```python
from build123d import *

# Parameters (mm, degrees)
SKETCH1_W           = 16
SKETCH1_H           = 20
BOSS_EXTRUDE1_DEPTH = 1.8
SKETCH2_W           = 16
SKETCH2_H           = 18.2
BOSS_EXTRUDE2_DEPTH = 1.8
SKETCH3_R           = 2.6
CUT_EXTRUDE1_DEPTH  = 1.8
SKETCH4_R           = 2.6
CUT_EXTRUDE2_DEPTH  = 1.8
FILLET1_R           = 2


with BuildPart() as part:
    # Sketch1 → Boss-Extrude1 (new body)
    with BuildSketch(Plane.XY):
        with Locations((8, 10)):
            Rectangle(SKETCH1_W, SKETCH1_H)
    extrude(amount=BOSS_EXTRUDE1_DEPTH)

    # Sketch2 → Boss-Extrude2 (add)
    with BuildSketch(Plane.XZ):
        with Locations((8, 10.9)):
            Rectangle(SKETCH2_W, SKETCH2_H)
    extrude(amount=-BOSS_EXTRUDE2_DEPTH)

    # Sketch3 → Cut-Extrude1 (cut)
    with BuildSketch(Plane.XY.offset(1.8)):
        with Locations((8, 10.8)):
            Circle(SKETCH3_R)
    extrude(amount=-CUT_EXTRUDE1_DEPTH, mode=Mode.SUBTRACT)

    # Sketch4 → Cut-Extrude2 (cut)
    with BuildSketch(Plane(origin=(0, 1.8, 0), x_dir=(1, 0, 0), z_dir=(0, 1, 0))):
        with Locations(Location((8, -10.8, 0), (0, 0, 270))):
            Circle(SKETCH4_R)
    extrude(amount=-CUT_EXTRUDE2_DEPTH, mode=Mode.SUBTRACT)

    # Fillet1
    fillet1_edges = [part.edges().sort_by_distance(p)[0] for p in [
        (8, 1.8, 1.8),
    ]]
    fillet(fillet1_edges, radius=FILLET1_R)


solid = part.part
```
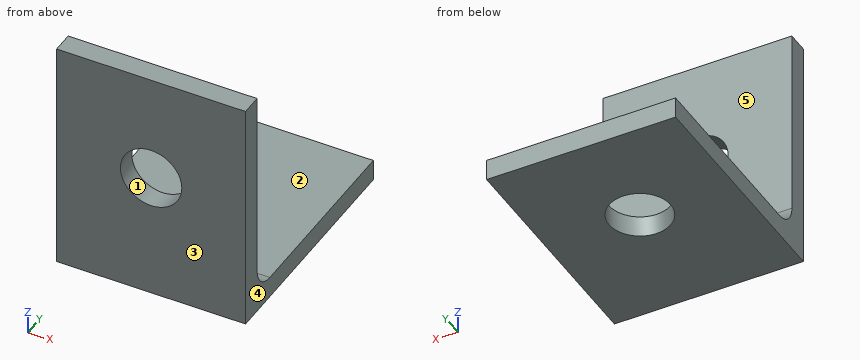
Check sheet for the modelled part. Datum: model origin and axes. Units: mm. Face numbers are marked on the shaded views. A direction names the side the tool comes from. Round coordinates to 2 decimals unless told otherwise and drop trailing zeros. Loops run counter-clockwise (first coordinate to the right, second up) from the corner with the lowest first, then second, coordinate; pieces in that order, holes last. Notation, with made-up numbers: (-35.75, 77.5) - (6.25, 77.5) arc R24 ccw to (6.25, 87.5) - close; hole circle Ø9 at (54, 25). An arc over 180 degrees is marked (long way). Answer as a JSON object with one key per item and string values. Group by question number.
Q1. Sectioned sample at A-A, the plane x = 8. Enter the section's corners in (y, z).
Q2. Sectioned sample at B-B, the plane z = 10.8. Enter the section's corners in (x, y), plus the area to 3 significant figures.
Q3. Sectioned sample at D-D, the plane x = 15.25. Enter the section's corners in (y, z).
Q4. Mould release check, pull along Z, two halves, no side actions. Record for the marked faces 1, 2 and 3: released by +Z, released by -Z, zero draft, split by the parting line, or undercut.
Q5. Gauge pin test, flat ends, axial feed: P1, Ø5, axis at x = 14, y = 7, coming from the +Z side; P2, Ø4.5, axis at x = 8, y = 10.8, coming from the +Z side. Record the tip position at first contact, or that the pin passes through.
Q6. Scan lines: line 1 along Y through (x, z) = (8, 1.3); line 2 along Z through (x, y) = (10.5, 4.5). Record each from-to range of solid material in increasing order. Write a range as [from, to].
Q7. Set-up check for the marked faces 4 and 5: record each of +Z, -Z, +X, -X, +Y, -Y from which the full face is reachable in a straight line by a thin tool's end or side.
Solution:
{
 "1": {"outline": "(0, 0) - (8.2, 0) - (8.2, 1.8) - (3.8, 1.8) arc R2 cw to (1.8, 3.8) - (1.8, 8.2) - (0, 8.2) - close; (0, 13.4) - (1.8, 13.4) - (1.8, 20) - (0, 20) - close; (13.4, 0) - (20, 0) - (20, 1.8) - (13.4, 1.8) - close"},
 "2": {"outline": "(0, 0) - (5.4, 0) - (5.4, 1.8) - (0, 1.8) - close; (10.6, 0) - (16, 0) - (16, 1.8) - (10.6, 1.8) - close", "area": "19.4 mm²"},
 "3": {"outline": "(0, 0) - (20, 0) - (20, 1.8) - (3.8, 1.8) arc R2 cw to (1.8, 3.8) - (1.8, 20) - (0, 20) - close"},
 "4": {"face 1": "undercut", "face 2": "released by +Z", "face 3": "zero draft"},
 "5": {"P1": "stops at z = 1.8", "P2": "passes through"},
 "6": {"line 1": "y = [0, 8.2], [13.4, 20]", "line 2": "z = [0, 1.8]"},
 "7": {"face 4": "+Z, -Z, +X, +Y, -Y", "face 5": "+Z, +X, -X, +Y"}
}
